Read the model definition and answer for the solid it produces. Units are mm, in the model's axes. Round coordinates to 2 decimals unless told otherwise and drop trailing zeros. Order: outer loops, then holes, each group sorted by start corner. A loop starts at its lowest first (then second) coordinate and runs counter-clockwise, first axis right, second up. Notation, with made-up numbers: (5.25, -31.5) -> (51.25, -31.5) arc R13 cw to (51.25, -8.5) -> close; hole circle Ø8 at (27.5, 55.5). An arc over 180 degrees is marked (long way). Use a Markdown table: item, result. Add a question column.
1. Consider L1, parallel to Z at x = -103.5, y = 1.5; L2, parallel to Z at x = -56, y = 2.25; L3, parallel to X at y = 5.5, z = 2161.5. Determine where each line is inside the solid, lowest interval first. Write a range as [from, to].
2. Section B-B, the plane y = 3.75 is taken. Give the vertices of the cut face in (x, z).
3. Given pin 1 (4 mm diameter, centred on y = 1.5, z = 2135.5, fed in from -X); pin 2 (4 mm diameter, centred on x = 318.5, y = 6.5, fed in from +Z); pin 3 (5 mm diameter, centred on x = 158.5, y = 7, fed in from -Z), each flat-ended and moving along its own axis, determine where each tip first touches the part or whether it passes through.
4. Section A-A, the plane x = 153 is taken. Give the vertices of the cut face in (y, z), then the cut area to 3 significant figures.
5. Section C-C, the plane z = 2119 is taken. Give the vertices of the cut face in (x, y), then the cut area to 3 significant figures.
```python
from build123d import *

# Parameters (mm, degrees)
EXTRUDE039434_DEPTH = 500


with BuildPart() as extrude039434_internal_superior:
    # Sketch223 (on Sketch) → Extrude039434 (new body, symmetric)
    with BuildSketch(Plane.XZ):
        Polygon((-600, 2300), (600, 2300), (200, 1900), (-200, 1900), align=None)
    extrude(amount=EXTRUDE039434_DEPTH, both=True)


with BuildPart() as internal_trim_horizontal:
    # Sweep012: sweep along a path in Sketch195
    with BuildLine(Plane.XZ) as sweep012_path:
        Line((-400, 2100), (-400, 0))
        Line((-400, 0), (400, 0))
        Line((400, 0), (400, 2100))
        Line((400, 2100), (-400, 2100))
    # Clone2D028 (on Sketch) → Sweep012 (sweep)
    with BuildSketch(Plane.ZY):
        with BuildLine():
            Line((-61.571224, 10), (-5.678418, 7))
            ThreePointArc((-5.678418, 7), (-1.645147, 5.136003), (0, 1.008624))
            Line((0, 1.008624), (0, 0))
            Line((0, 0), (-70, 0))
            Line((-70, 0), (-70, 2.011499))
            ThreePointArc((-70, 2.011499), (-67.503171, 7.81797), (-61.571224, 10))
        make_face()
    sweep(path=sweep012_path.line, is_frenet=True, transition=Transition.RIGHT)

    # Common001: intersect Extrude039434_Internal_superior_
    add(extrude039434_internal_superior.part, mode=Mode.INTERSECT)


solid = internal_trim_horizontal.part
```
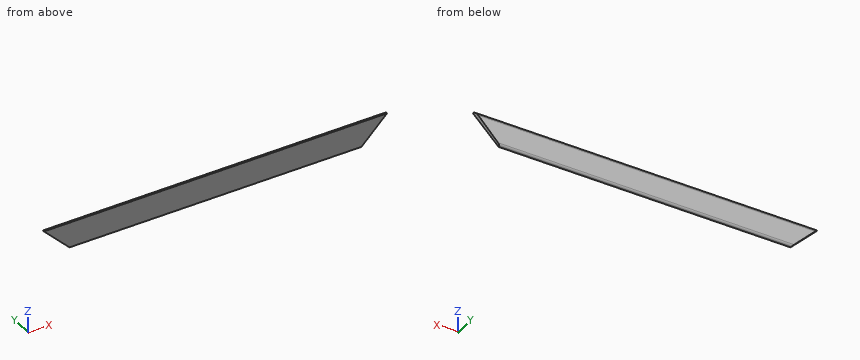
Verdict:
| question | item | result |
|---|---|---|
| 1 | L1 | z = [2100.02, 2170] |
| 1 | L2 | z = [2100.13, 2170] |
| 1 | L3 | x = [-461.5, 461.5] |
| 2 | outline | (-469.81, 2169.81) -> (-400.66, 2100.66) -> (400.66, 2100.66) -> (469.81, 2169.81) -> close |
| 3 | pin 1 | stops at x = -437.5 |
| 3 | pin 2 | stops at z = 2169.6 |
| 3 | pin 3 | stops at z = 2101.12 |
| 4 | outline | (0, 2100) -> (1.01, 2100) arc R6 ccw to (7, 2105.68) -> (10, 2161.57) arc R8 ccw to (2.01, 2170) -> (0, 2170) -> close |
| 4 | area | 578 mm2 |
| 5 | outline | (-419, 0) -> (419, 0) -> (419, 7.72) -> (-419, 7.72) -> close |
| 5 | area | 6,470 mm2 |
